from build123d import *

# Parameters (mm, degrees)
SKETCH1_R           = 3.75
BOSS_EXTRUDE1_DEPTH = 3.5
CUT_EXTRUDE1_DEPTH  = 1.75
BOSS_EXTRUDE3_DEPTH = 80
SKETCH9_R           = 2
CUT_EXTRUDE3_DEPTH  = 7
FILLET2_R           = 2
BOSS_EXTRUDE7_DEPTH = 3.5


with BuildPart() as part:
    # Sketch1 → Boss-Extrude1 (new body, symmetric)
    with BuildSketch(Plane(origin=(0, 0, 0), x_dir=(0, 0, -1), z_dir=(1, 0, 0))):
        with BuildLine():
            Line((-80.521669114, -9.954039671), (-3.96947016, -18))
            ThreePointArc((-3.96947016, -18), (6.057083574, -10.773431066), (0, 0))
            Line((0, 0), (-80, 0))
            ThreePointArc((-80, 0), (-84.983850029, -4.729497083), (-80.521669114, -9.954039671))
        make_face()
        with Locations((-2, -11)):
            Circle(SKETCH1_R, mode=Mode.SUBTRACT)
        Polygon((-53.094727027, -18.903008846), (-49, -13.267100598), (-55, -12.636475186), (-55.630625412, -18.636475186), align=None)
    extrude(amount=BOSS_EXTRUDE1_DEPTH, both=True)

    # Sketch6 → Cut-Extrude1 (cut, symmetric)
    with BuildSketch(Plane(origin=(0, 0, 0), x_dir=(0, 0, -1), z_dir=(1, 0, 0))):
        with BuildLine():
            ThreePointArc((1.619477331, -11.980756773), (-4.659098946, -13.644180931), (-2.960378385, -7.375062296))
            Line((-2.960378385, -7.375062296), (-31.959880017, -15.058089377))
            Line((-31.959880017, -15.058089377), (-3.96947016, -18))
            ThreePointArc((-3.96947016, -18), (0.558835237, -17.340846662), (4.220806393, -14.596762087))
            Line((4.220806393, -14.596762087), (1.619477331, -11.980756773))
        make_face()
    extrude(amount=CUT_EXTRUDE1_DEPTH, both=True, mode=Mode.SUBTRACT)

    # Sketch8 → Boss-Extrude3 (add)
    with BuildSketch(Plane.XY):
        with BuildLine():
            Line((-3.5, 0), (3.5, 0))
            ThreePointArc((3.5, 0), (0, 0.120714291), (-3.5, 0))
        make_face()
    extrude(amount=BOSS_EXTRUDE3_DEPTH)

    # Sketch9 → Cut-Extrude3 (cut)
    with BuildSketch(Plane(origin=(0, 5.579502847, 53.085423559), x_dir=(1, 0, 0), z_dir=(0, 0.104528463, 0.994521895))):
        with Locations((0, -21.34936641)):
            Circle(SKETCH9_R)
    extrude(amount=-CUT_EXTRUDE3_DEPTH, mode=Mode.SUBTRACT)

    # Fillet2
    fillet2_edges = [part.edges().sort_by_distance(p)[0] for p in [
        (-3.5, -18.769742016, 54.362676219),
        (3.5, -18.769742016, 54.362676219),
    ]]
    fillet(fillet2_edges, radius=FILLET2_R)

    # Sketch10 → Boss-Extrude7 (add)
    with BuildSketch(Plane.ZY.offset(-1.75)):
        Polygon((31.959880017, -15.058089377), (30.04729926, -14.551376885), (16.886307052, -15.934652906), (16.959880017, -16.634652906), align=None)
        Polygon((31.959880017, -15.058089377), (31.886307052, -14.358089377), (30.04729926, -14.551376885), align=None)
    extrude(amount=BOSS_EXTRUDE7_DEPTH)


solid = part.part
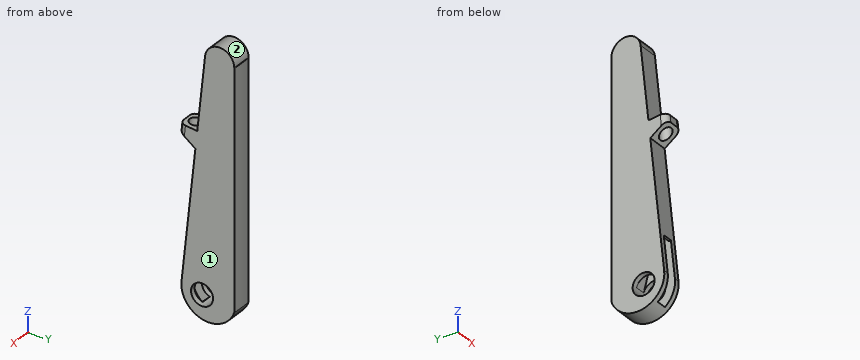
Design review of the part built by this model. Coordinates are the model's own, in mm. Face numbers are marked on the shaded views. Give positions to 0.01 mm unless a question says otherwise; leave off trailing zeros. Loops run counter-clockwise (first coordinate to the right, second up) from the corner with the lowest first, then second, coordinate; pieces in that order, holes last. Notation, with made-up numbers: M 43.5,-39.75 L 49.5,-39.75 A9 ccw 49.5,-24.75 Z; hole C 44.5,76 d11. An arc over 180 degrees is marked long. One line per question, with ' | ' between items. Start each with the question number.
1. Add section B-B (z = 2). Write out the cut boundary in (x, y).
2. Insertion check: P1, Ø1.5, axis at x = 2.5, y = -7, coming from the -Z side; P2, Ø1, axis at x = -0.5, y = -3.5, coming from the -Z side. Each pin has a flat end and moves straight along its axis. Give the tip position at first contact, or say it passes through.
3. The part is to be moulded in two halves that separate along Z. For the marked faces 1 and 2, say which applies: released by +Z, released by -Z, zero draft, split by the parting line, or undercut.
4. To check wall thickness, follow L1, parallel to Y at x = 0.25, z = 2; L2, parallel to Z at x = 1.75, y = -5.5; L3, parallel to Z at x = 0, y = -6. State the ranges of each line that lie inside material, in increasing order.
5. Add section A-A (x = 0.25). Write out the cut boundary in (y, z), plus the area to 3 significant figures.
6. Add section C-C (y = -8.25). Write out the cut boundary in (x, z), plus the area to 3 significant figures.
7. Add section D-D (z = 23). Write out the cut boundary in (x, y), plus the area to 3 significant figures.
Worked out:
1) outline: M -3.5,-18 L -1.75,-18 L -1.75,-14.75 L -3.5,-14.75 Z; M -3.5,-7.25 L 3.5,-7.25 L 3.5,0 A50.8 ccw -3.5,0 Z; M 1.75,-18 L 3.5,-18 L 3.5,-14.75 L 1.75,-14.75 Z
2) P1: stops at z = -6.22 | P2: stops at z = -4.95
3) face 1: zero draft | face 2: released by +Z
4) L1: y = -7.25 to 0.12 | L2: z = -5.68 to 84.96 | L3: z = -5.85 to 84.89
5) outline: M -18.9,53.09 L -17.95,52.41 L -17.63,55.52 L -18.64,55.63 Z; M -16.63,16.96 L -15.93,16.89 L -14.55,30.05 L -7.38,2.96 A3.75 cw -11.98,-1.62 L -14.6,-4.22 A9.27 ccw 0,0 L 0.12,0 L 0.12,80 L 0,80 A4.99 ccw -9.95,80.52 L -12.64,55 L -13.68,55.11 L -14.25,49.71 L -13.27,49 Z | area: 1,080 mm²
6) outline: M -3.5,-6.26 L 3.5,-6.26 L 3.5,-0.55 L -3.5,-0.55 Z; M -3.5,4.55 L -1.75,4.55 L -1.75,6.26 L 1.75,6.26 L 1.75,4.55 L 3.5,4.55 L 3.5,83.78 L -3.5,83.78 Z | area: 589 mm²
7) outline: M -3.5,-16 L 3.5,-16 L 3.5,0 A50.8 ccw -3.5,0 Z; hole M -1.75,-15.29 L 1.75,-15.29 L 1.75,-12.68 L -1.75,-12.68 Z | area: 103 mm²
